Input: dimensioned drawing with shaded views. Units: mm. Origin: part minimum x, y, z. Round coordinates to 2 decimals unless told otherwise and drop trailing zeros. Loops run counter-clockwise (first coordinate to the right, second up) from the corner with the lowest first, then second, coordinate; pieces in that order, holes last. Notation, with made-up numbers: (2, 88.5) - (54, 88.5) arc R24 ccw to (54, 113.5) - close; hole circle Ø5 at (-28, -35). An arc over 180 degrees is marked (long way). One line per question, with ' | ' between items. Start each with the question number.
Item 1: Section C-C, the plane x = 90. Return loops of the section in (y, z).
Item 2: First-contact query: pin 1 (1.5 mm diameter, centred on y = 14.5, z = 1, fed in from -X); pin 2 (0.9 mm diameter, centred on x = 92, z = 2, fed in from -Y). Flat tips, straight axial feed; report the tip coordinate or a pass-through.
Item 3: Section B-B, the plane z = 1.65. Return loops of the section in (x, y), plus the area to 3 significant figures.
Item 4: Section A-A, the plane y = 21. Return loops of the section in (x, z), plus the area to 3 significant figures.
Item 5: Material intervals for line 1 along X through (y, z) = (20.75, 2.2); line 2 along Y through (x, z) = (11.5, 0.9); line 3 along X through (y, z) = (18.25, 1.25), sorted ascending.
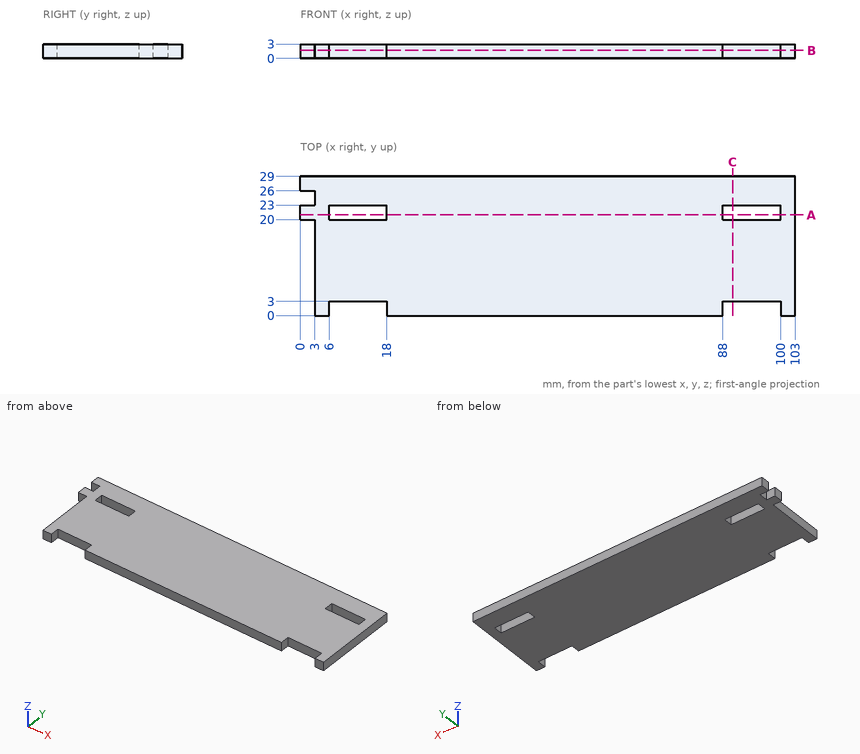
Return value:
1) outline: (3, 0) - (20, 0) - (20, 3) - (3, 3) - close; (23, 0) - (29, 0) - (29, 3) - (23, 3) - close
2) pin 1: x = 3 | pin 2: y = 3
3) outline: (0, 20) - (3, 20) - (3, 0) - (6, 0) - (6, 3) - (18, 3) - (18, 0) - (88, 0) - (88, 3) - (100, 3) - (100, 0) - (103, 0) - (103, 29) - (0, 29) - (0, 26) - (3, 26) - (3, 23) - (0, 23) - close; hole (6, 20) - (18, 20) - (18, 23) - (6, 23) - close; hole (88, 20) - (100, 20) - (100, 23) - (88, 23) - close | area: 2,770 mm2
4) outline: (0, 0) - (6, 0) - (6, 3) - (0, 3) - close; (18, 0) - (88, 0) - (88, 3) - (18, 3) - close; (100, 0) - (103, 0) - (103, 3) - (100, 3) - close | area: 237 mm2
5) line 1: 0 to 6, 18 to 88, 100 to 103 | line 2: 3 to 20, 23 to 29 | line 3: 3 to 103
